Design review of the part shown in the three views and the two pictorial views. Dimensions are in mm from the part's minimum x, y and z. Give positions to 0.01 mm unless a question says otherwise; leave off trailing zeros. Order: outer loops, then holes, each group sorted by start corner. A loop starts at its lowest first (then second) coordinate and runs counter-clockwise, first axis right, second up. Notation, with made-up numbers: (0, -8.75) - (5, -8.75) arc R27 cw to (5, 21.25) - close; hole circle Ø11 at (-25, -18.5). An arc over 180 degrees is marked (long way). Put each result on its own line as item: value.
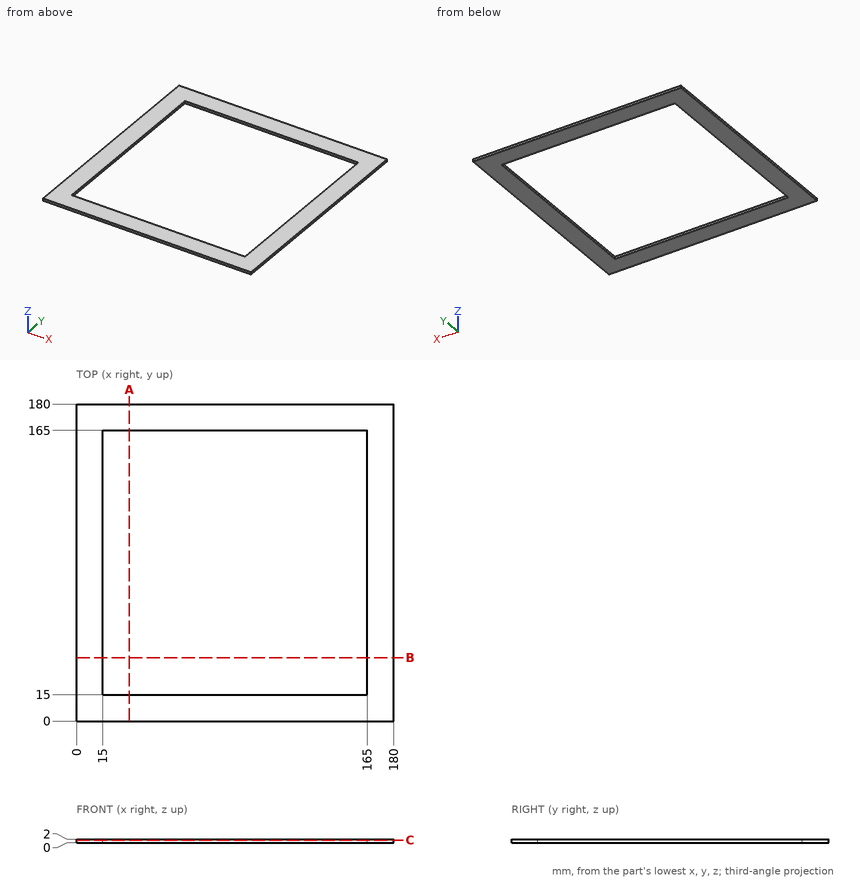
(1) Wall thickness on L1, parallel to X at y = 133.5, z = 1.4: over which ranges is the line inside the solid? List them lowest first.
The answers:
L1: 0 to 15, 165 to 180
(2) Take a section at C-C, the plane z = 1.4. Write out the cut boundary in (x, y).
The answers:
outline: (0, 0) - (180, 0) - (180, 180) - (0, 180) - close; hole (15, 15) - (165, 15) - (165, 165) - (15, 165) - close
(3) Take a section at A-A, the plane x = 30. Write out the cut boundary in (y, z), then the cut area to 3 significant figures.
The answers:
outline: (0, 0) - (15, 0) - (15, 2) - (0, 2) - close; (165, 0) - (180, 0) - (180, 2) - (165, 2) - close
area: 60.0 mm^2
(4) Clearance check with a flat-ended pin moving along its axis: pin 1 Ø0.6 at (y, z) = (90, 1) entering from -X. State where the tip first meets the part, or that it passes through.
The answers:
pin 1: x = 0
